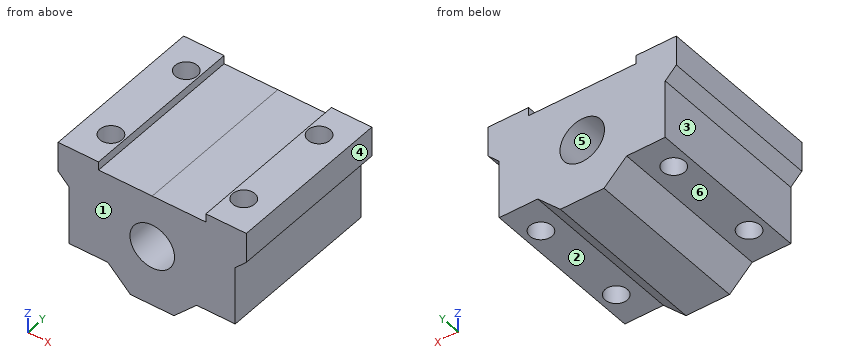
```python
from build123d import *

# Parameters (mm, degrees)
F0_R          = 4.025
F1_DEPTH      = 30
F2_R          = 2
F3_DEPTH      = 10.9999993406
F3_DEPTH_BACK = 25


# Not quite as in the source:
# - ends of sketch curves that miss each other by under 0.0002 mm in the source are joined


with BuildPart() as f1:
    # F0 (on Front) → F1 (new body)
    with BuildSketch(Plane.XZ):
        Polygon((-17, 10.9999990659), (-17, 5.5723366328), (-15, 3.5723366328), (-15, -7.0000008242), (-8.0288857139, -7.0000004412), (-3.9351008678, -11.0000002162), (3.022e-07, -11), (3.9351014722, -10.9999997838), (8.0288857139, -7.0000004412), (15, -7.0000008242), (15, 3.5723366328), (17, 5.5723366328), (17, 10.9999990659), (9.6955373869, 10.9999994673), (9.6955373029, 9.4717088947), (8.4e-08, 9.4717094274), (-9.6955373029, 9.4717088947), (-9.6955373869, 10.9999994673), align=None)
        Circle(F0_R, mode=Mode.SUBTRACT)
    extrude(amount=F1_DEPTH)

    # F2 (on Top) → F3 (cut, two sides)
    with BuildSketch(Plane.XY) as f3_sk:
        with Locations((-12, -6)):
            Circle(F2_R)
        with Locations((-12, -24)):
            Circle(F2_R)
        with Locations((12, -6)):
            Circle(F2_R)
        with Locations((12, -24)):
            Circle(F2_R)
    extrude(amount=F3_DEPTH, mode=Mode.SUBTRACT)
    extrude(f3_sk.sketch, amount=-F3_DEPTH_BACK, mode=Mode.SUBTRACT)


solid = f1.part
```
Verification items for the finished model (mm, model axes). Face numbers are marked on the shaded views. A direction names the side the tool comes from. Give positions to 0.01 mm unless a question says otherwise; leave off trailing zeros. Loops run counter-clockwise (first coordinate to the right, second up) from the corner with the lowest first, then second, coordinate; pieces in that order, holes last.
1. Section check A-A, the plane y = -24. Enter the section's corners in (x, z) (3 decimals).
2. Thickness scan on line 1 (Y direction, x = 12, z = -2); line 2 (X direction, y = -6.5, z = 1); line 3 (Y direction, x = -11.5, z = 2.5). Record the ranges inside material, lowest first.
3. Section check B-B, the plane x = 12. Enter the section's corners in (y, z).
4. Mould release check, pull along X, two halves, no side actions. Record for the marked faces 4, 5 and 6: released by +X, released by -X, zero draft, split by the parting line, or undercut.
5. Section check D-D, the plane y = -15. Enter the section's corners in (x, z) (3 decimals), then the cut area to 3 significant figures.
6. Set-up check for the marked faces 1, 2 and 3: record each of +Z, -Z, +X, -X, +Y, -Y from which the full face is reachable in a straight line by a thin tool's end or side.
7. Section check C-C, the plane x = -2. Enter the section's corners in (y, z).
8. Go/stop test with flat-tipped pins: pin 1 Ø6 at (x, y) = (-10, -21) entering from -Z; pin 2 Ø5 at (x, y) = (2.5, -21) entering from +Z; pin 3 Ø5.5 at (x, y) = (11, -17) entering from -Z. Record where each tip stops, or that it passes through.
Geometry says:
1. outline: (-17, 5.572) - (-15, 3.572) - (-15, -7) - (-14, -7) - (-14, 11) - (-17, 11) - close; (-10, -7) - (-8.029, -7) - (-3.935, -11) - (3.935, -11) - (8.029, -7) - (10, -7) - (10, 11) - (9.696, 11) - (9.696, 9.472) - (0, 9.472) - (-9.696, 9.472) - (-9.696, 11) - (-10, 11) - close; (14, -7) - (15, -7) - (15, 3.572) - (17, 5.572) - (17, 11) - (14, 11) - close; hole circle Ø8.05 at (0, 0)
2. line 1: y = -30 to -26, -22 to -8, -4 to 0
2. line 2: x = -15 to -13.94, -10.06 to -3.9, 3.9 to 10.06, 13.94 to 15
2. line 3: y = -30 to -25.94, -22.06 to -7.94, -4.06 to 0
3. outline: (-30, -7) - (-26, -7) - (-26, 11) - (-30, 11) - close; (-22, -7) - (-8, -7) - (-8, 11) - (-22, 11) - close; (-4, -7) - (0, -7) - (0, 11) - (-4, 11) - close
4. face 4: released by +X
4. face 5: undercut
4. face 6: zero draft
5. outline: (-17, 5.572) - (-15, 3.572) - (-15, -7) - (-8.029, -7) - (-3.935, -11) - (3.935, -11) - (8.029, -7) - (15, -7) - (15, 3.572) - (17, 5.572) - (17, 11) - (9.696, 11) - (9.696, 9.472) - (0, 9.472) - (-9.696, 9.472) - (-9.696, 11) - (-17, 11) - close; hole circle Ø8.05 at (0, 0)
5. area: 533 mm2
6. face 1: +Z, -Z, +X, -X, -Y
6. face 2: -Z, +X, +Y, -Y
6. face 3: -Z, -X, +Y, -Y
7. outline: (-30, -11) - (0, -11) - (0, -3.49) - (-30, -3.49) - close; (-30, 3.49) - (0, 3.49) - (0, 9.47) - (-30, 9.47) - close
8. pin 1: stops at z = -8.01
8. pin 2: stops at z = 9.47
8. pin 3: stops at z = -7
